```python
from build123d import *

# Parameters (mm, degrees)
SKETCH2_R           = 22.86
BOSS_EXTRUDE1_DEPTH = 83.82
SKETCH3_R           = 27.94
BOSS_EXTRUDE2_DEPTH = 14.224
SKETCH4_R           = 7.493
BOSS_EXTRUDE3_DEPTH = 4.445
SKETCH5_R           = 29.337
BOSS_EXTRUDE4_DEPTH = 10.16
SKETCH6_R           = 25.4
BOSS_EXTRUDE5_DEPTH = 24.13
SKETCH7_R           = 21.209
BOSS_EXTRUDE6_DEPTH = 30.48
SKETCH8_R           = 14.478
BOSS_EXTRUDE7_DEPTH = 10.16
SKETCH9_R           = 10.9855
BOSS_EXTRUDE8_DEPTH = 3.556
SKETCH10_R          = 6.35
CUT_EXTRUDE1_DEPTH  = 25.4


with BuildPart() as part:
    # Sketch2 → Boss-Extrude1 (new body)
    with BuildSketch(Plane.XY):
        Circle(SKETCH2_R)
    extrude(amount=BOSS_EXTRUDE1_DEPTH)

    # Sketch3 → Boss-Extrude2 (add)
    with BuildSketch(Plane.XY.offset(83.82)):
        Circle(SKETCH3_R)
    extrude(amount=BOSS_EXTRUDE2_DEPTH)

    # Sketch4 → Boss-Extrude3 (add)
    with BuildSketch(Plane(origin=(0, 0, 0), x_dir=(-1, 0, 0), z_dir=(0, 0, -1))):
        Circle(SKETCH4_R)
    extrude(amount=BOSS_EXTRUDE3_DEPTH)

    # Sketch5 → Boss-Extrude4 (add)
    with BuildSketch(Plane.XY.offset(98.044)):
        Circle(SKETCH5_R)
    extrude(amount=BOSS_EXTRUDE4_DEPTH)

    # Sketch6 → Boss-Extrude5 (add)
    with BuildSketch(Plane.XY.offset(108.204)):
        with Locations(Location((0, 0, 0), (0, 0, 180))):
            Circle(SKETCH6_R)
    extrude(amount=BOSS_EXTRUDE5_DEPTH)

    # loft up to a face of the part (loft1)
    loft([Face(Wire([part.edges().sort_by_distance((-20.082558447, 21.385752623, 108.204))[0]])), Face(Wire([part.edges().sort_by_distance((17.387496491, -18.515803137, 132.334))[0]]))])

    # Sketch7 → Boss-Extrude6 (add)
    with BuildSketch(Plane.XY.offset(132.334)):
        with Locations(Location((0, 0, 0), (0, 0, 180))):
            Circle(SKETCH7_R)
    extrude(amount=BOSS_EXTRUDE6_DEPTH)

    # Sketch8 → Boss-Extrude7 (add)
    with BuildSketch(Plane.XY.offset(162.814)):
        Circle(SKETCH8_R)
    extrude(amount=BOSS_EXTRUDE7_DEPTH)

    # Sketch9 → Boss-Extrude8 (add)
    with BuildSketch(Plane.XY.offset(172.974)):
        Circle(SKETCH9_R)
    extrude(amount=BOSS_EXTRUDE8_DEPTH)

    # loft up to a face of the part (loft2)
    loft([Face(Wire([part.edges().sort_by_distance((14.51855957, -15.460695619, 162.814))[0]])), Face(Wire([part.edges().sort_by_distance((-9.910873, 10.554007788, 172.974))[0]]))])

    # Sketch10 → Cut-Extrude1 (cut)
    with BuildSketch(Plane.XY.offset(176.53)):
        Circle(SKETCH10_R)
    extrude(amount=-CUT_EXTRUDE1_DEPTH, mode=Mode.SUBTRACT)


solid = part.part
```
Model file for the job. Use its own axes, mm. A direction names the side the tool comes from. Coordinates: 2 decimals unless noted, no trailing zeros. Write each loop counter-clockwise with the first axis right and the second up, starting at its lowest first coordinate (ties: lowest second). Pieces come first, ordered by that corner, then holes. Notation, with made-up numbers: (48, 2.5) - (83, 2.5) arc R14 ccw to (83, 18.5) - close; hole circle Ø11 at (22.25, -16.5). An arc over 180 degrees is marked (long way). Use a Markdown table: item, result. Add a question column.
Item 1: 3-axis set-ups, long thin cutter, end or side, ignore diameter. For faces 1 (the face through (0, 0, -4.445)), 2 (the face through (21.804, 6.867, 41.323)), 3 (the face through (6, 21, 132.334)): which of +Z, -Z, +X, -X, +Y, -Y reach the whole face in a straight line?
Item 2: Two-plate mould, pull along Y, no slides. Class faces 4 (the face through (-2, 11, 172.974)), 5 (the face through (0.98, 7.43, -2.19)), 6 (the face through (-1.38, -6.2, 164.01)): pulls with the +Y half, pulls with the -Y half, needs draft (parallel to the pull), parting line crosses it, or undercut.
Item 3: Drop flat-ended pins along their axis: pin 1 (1.5 mm diameter, centred on x = 17, y = -5, fed in from +Z); pin 2 (6.5 mm diameter, centred on x = 1.5, y = -0.5, fed in from +Z); pin 3 (3 mm diameter, centred on y = 12.5, z = 126.5, fed in from -X). Give the stop position or say it passes through.
Item 4: Drill centre lines: line 1 along Y through (x, z) = (0, 157.5); line 2 along Z through (x, y) = (9, -4); line 3 along Z through (x, y) = (-19, -13). Where is each one in solid material? Low to high.
Item 5: Band-saw the part on B-B, the plane z = 12. Write the cut outline in (x, y).
A:
| question | item | result |
|---|---|---|
| 1 | face 1 | -Z, +X, -X, +Y, -Y |
| 1 | face 2 | -Z |
| 1 | face 3 | +Z |
| 2 | face 4 | needs draft |
| 2 | face 5 | parting line crosses it |
| 2 | face 6 | undercut |
| 3 | pin 1 | stops at z = 169.21 |
| 3 | pin 2 | stops at z = 151.13 |
| 3 | pin 3 | stops at x = -24 |
| 4 | line 1 | y = -21.21 to -6.35, 6.35 to 21.21 |
| 4 | line 2 | z = 0 to 176.53 |
| 4 | line 3 | z = 83.82 to 132.33 |
| 5 | outline | circle Ø45.72 at (0, 0) |
